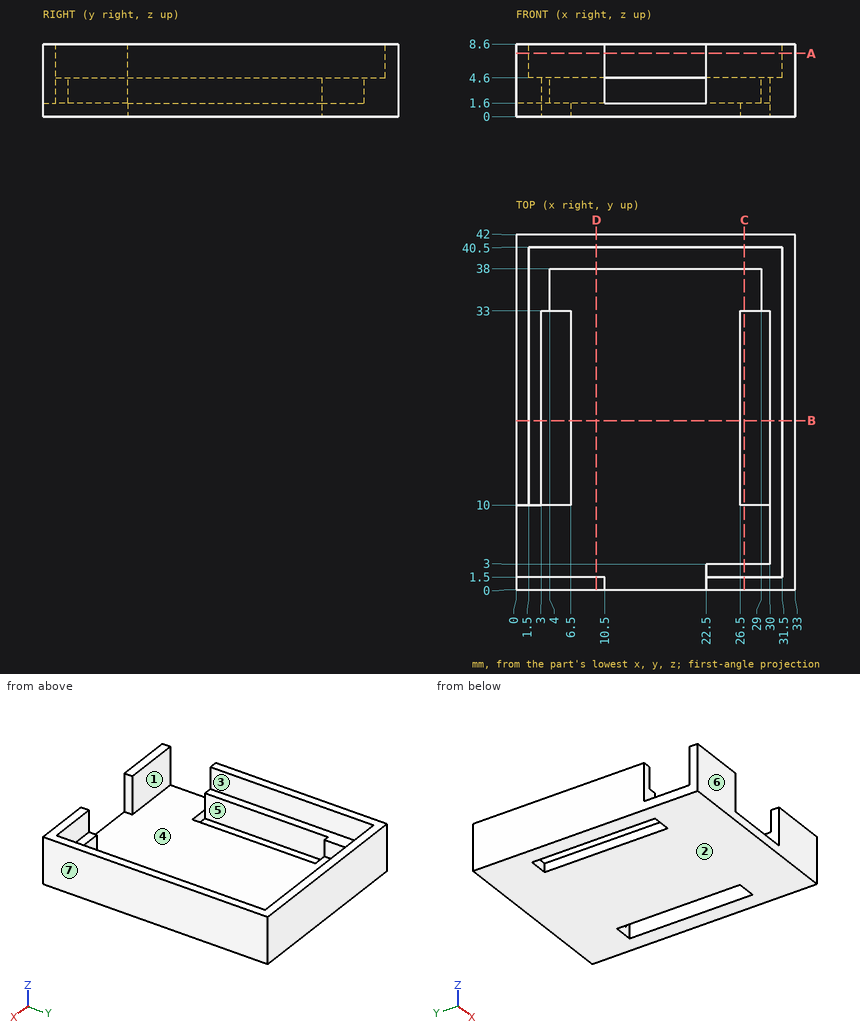
Design review of the part shown in the three views and the two pictorial views. Dimensions are in mm from the part's minimum x, y and z. A direction names the side the tool comes from. Give positions to 0.01 mm unless a question says otherwise; leave off trailing zeros. Write each loop counter-clockwise with the first axis right and the second up, starting at its lowest first coordinate (ties: lowest second). Pieces come first, ordered by that corner, then holes.
Item 1: Machinability: for the marked faces 1, 2 and 3, which of the approach directions +Z, -Z, +X, -X, +Y, -Y give a long, thin tool a straight path to every point of the face, cutting with its end or side? Answer none if there is none.
Item 2: Take a section at A-A (z = 7.5). Give the boundary of the cut face in (x, y), and give its area (3 significant figures).
Item 3: Take a section at C-C (x = 27). Give the boundary of the cut face in (y, z).
Item 4: Take a section at D-D (x = 9.5). Give the boundary of the cut face in (y, z), and give its area (3 significant figures).
Item 5: Insertion check: P1, Ø1.2, axis at y = 21, z = 7.5, coming from the -X side; P2, Ø1.5, axis at x = 12.5, y = 26.5, coming from the +Z side. Each pin has a flat end and moves straight along its axis. Give the tip position at first contact, or say it passes through.
Item 6: The part is to be moulded in two halves that separate along Y. For the marked faces 4, 5, 6 and 7, say which applies: +Y half, -Y half, draft (parallel to the pull), parting line (faces both ways), or undercut.
Item 7: Take a section at B-B (y = 20). Give the boundary of the cut face in (x, z).
Item 8: Wall thickness on probe 1 along X at (y, z) = (19.5, 4); probe 2 along Y at (x, z) = (4.5, 3.25); probe 3 along Y at (x, z) = (29.5, 4.5): over which ranges is each line inside the solid? List them lowest first.
Established:
1. face 1: +Z, -X
1. face 2: -Z, +X, -X, +Y, -Y
1. face 3: +Z
2. outline: (0, 0) - (10.5, 0) - (10.5, 1.5) - (0, 1.5) - close; (0, 10) - (1.5, 10) - (1.5, 40.5) - (31.5, 40.5) - (31.5, 1.5) - (22.5, 1.5) - (22.5, 0) - (33, 0) - (33, 42) - (0, 42) - close
2. area: 185 mm2
3. outline: (0, 0) - (10, 0) - (10, 1.6) - (3, 1.6) - (3, 4.6) - (1.5, 4.6) - (1.5, 8.6) - (0, 8.6) - close; (33, 0) - (42, 0) - (42, 8.6) - (40.5, 8.6) - (40.5, 4.6) - (38, 4.6) - (38, 1.6) - (33, 1.6) - close
4. outline: (0, 0) - (42, 0) - (42, 8.6) - (40.5, 8.6) - (40.5, 4.6) - (38, 4.6) - (38, 1.6) - (1.5, 1.6) - (1.5, 8.6) - (0, 8.6) - close
4. area: 95.7 mm2
5. P1: stops at x = 0
5. P2: stops at z = 1.6
6. face 4: undercut
6. face 5: undercut
6. face 6: -Y half
6. face 7: draft
7. outline: (0, 0) - (3, 0) - (3, 4.6) - (1.5, 4.6) - (1.5, 8.6) - (0, 8.6) - close; (6.5, 0) - (26.5, 0) - (26.5, 1.6) - (6.5, 1.6) - close; (30, 0) - (33, 0) - (33, 8.6) - (31.5, 8.6) - (31.5, 4.6) - (30, 4.6) - close
8. probe 1: x = 0 to 3, 30 to 33
8. probe 2: y = 0 to 1.5, 38 to 42
8. probe 3: y = 0 to 3, 33 to 42
